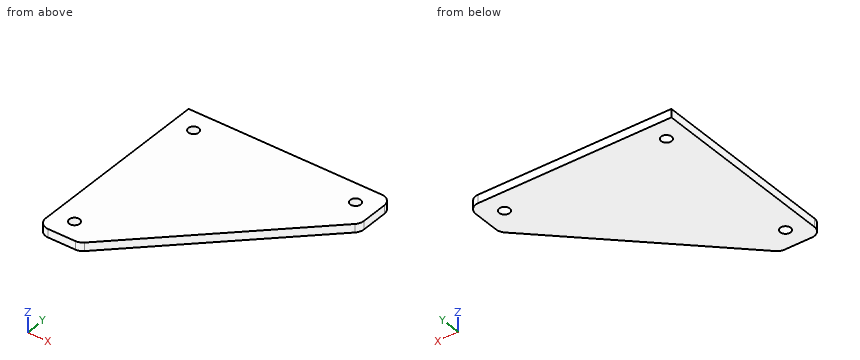
from build123d import *

# Parameters (mm, degrees)
BOSS_EXTRU_1_DEPTH      = 4
ESQUISSE2_R             = 2.5
ENL_V_MAT_EXTRU_1_DEPTH = 4
CONG_1_R                = 5


with BuildPart() as part:
    # Esquisse1 → Boss.-Extru.1 (new body)
    with BuildSketch(Plane.XY):
        Polygon((-46.45758945, 41.15105452), (51.118168125, 41.15105452), (51.118168125, 21.15105452), (-26.45758945, -53.798440429), (-46.45758945, -53.798440429), align=None)
    extrude(amount=BOSS_EXTRU_1_DEPTH)

    # Esquisse2 → Enlèv. mat.-Extru.1 (cut)
    with BuildSketch(Plane.XY.offset(4)):
        with Locations((-36.45758945, 31.15105452)):
            Circle(ESQUISSE2_R)
        with Locations((41.118168125, 31.15105452)):
            Circle(ESQUISSE2_R)
        with Locations((-36.45758945, -43.798440429)):
            Circle(ESQUISSE2_R)
    extrude(amount=-ENL_V_MAT_EXTRU_1_DEPTH, mode=Mode.SUBTRACT)

    # Congé1
    cong_1_edges = [part.edges().sort_by_distance(p)[0] for p in [
        (51.118168125, 41.15105452, 2),
        (51.118168125, 21.15105452, 2),
        (-26.45758945, -53.798440429, 2),
        (-46.45758945, -53.798440429, 2),
    ]]
    fillet(cong_1_edges, radius=CONG_1_R)


solid = part.part
Can you work these out from the model? Positions are in its coordinate system, mm. Give positions to 0.01 mm unless a question says otherwise; leave off trailing zeros. Loops run counter-clockwise (first coordinate to the right, second up) from the corner with the lowest first, then second, coordinate; pieces in that order, holes last. Notation, with made-up numbers: (64.5, -35.5) - (74.5, -35.5) arc R17 cw to (74.5, -2.5) - close; hole circle Ø10 at (-21, 67.5). An arc over 180 degrees is marked (long way). Answer as a JSON object with one key per item and string values.
Q1. Imagine slicing it at A-A on z = 0.95. Write out the boundary of the cut face in (x, y).
Geometry says:
{"outline": "(-46.46, -48.8) arc R5 ccw to (-41.46, -53.8) - (-28.48, -53.8) arc R5 ccw to (-25, -52.39) - (49.59, 19.68) arc R5 ccw to (51.12, 23.27) - (51.12, 36.15) arc R5 ccw to (46.12, 41.15) - (-46.46, 41.15) - close; hole circle Ø5 at (-36.46, -43.8); hole circle Ø5 at (-36.46, 31.15); hole circle Ø5 at (41.12, 31.15)"}
Q2. If I drill on L1, parallel to X at y = 32.5, z = 2.5; L2, parallel to Y at x = 39, z = 3.5; L3, parallel to Y at x = -28, z = 0.6, over which ranges is the centre line in solid material (lowest first)?
Geometry says:
{"L1": "-46.46 to -38.56, -34.35 to 39.01, 43.22 to 51.12", "L2": "9.44 to 29.82, 32.48 to 41.15", "L3": "-53.78 to 41.15"}
Q3. Imagine slicing it at C-C on y = -38.5. Write out the boundary of the cut face in (x, z).
Geometry says:
{"outline": "(-46.46, 0) - (-10.62, 0) - (-10.62, 4) - (-46.46, 4) - close"}
Q4. Imagine slicing it at D-D on x = 11. Write out the boundary of the cut face in (y, z).
Geometry says:
{"outline": "(-17.61, 0) - (41.15, 0) - (41.15, 4) - (-17.61, 4) - close"}
Q5. Imagine slicing it at B-B on x = 40. Write out the boundary of the cut face in (y, z), plus the area to 3 significant figures.
Geometry says:
{"outline": "(10.41, 0) - (28.92, 0) - (28.92, 4) - (10.41, 4) - close; (33.39, 0) - (41.15, 0) - (41.15, 4) - (33.39, 4) - close", "area": "105 mm²"}
